CAD build for the part. Positions are in the model's coordinates, mm. Give positions to 0.01 mm unless a question says otherwise; leave off trailing zeros.
```python
from build123d import *

# Parameters (mm, degrees)
BOSS_EXTRUDE1_DEPTH = 749.3
BOSS_EXTRUDE2_DEPTH = 12.7
SKETCH3_W           = 25.4
SKETCH3_H           = 12.7
CUT_EXTRUDE1_DEPTH  = 6.35
SKETCH4_R           = 1.5875
CUT_EXTRUDE2_DEPTH  = 70.358
SKETCH5_R           = 1.5875
CUT_EXTRUDE3_DEPTH  = 70.358


with BuildPart() as part:
    # Sketch1 → Boss-Extrude1 (new body)
    with BuildSketch(Plane.XY):
        Polygon((0, 11.1125), (1.5875, 12.7), (4.7625, 12.7), (6.35, 11.1125), (6.35, 1.5875), (4.7625, 0), (1.5875, 0), (0, 1.5875), align=None)
    extrude(amount=BOSS_EXTRUDE1_DEPTH)

    # Sketch2 → Boss-Extrude2 (add)
    with BuildSketch(Plane.XY.offset(749.3)):
        with BuildLine():
            Line((4.7625, 9.525), (4.7625, 3.175))
            ThreePointArc((4.7625, 3.175), (3.175, 1.5875), (1.5875, 3.175))
            Line((1.5875, 3.175), (1.5875, 9.525))
            ThreePointArc((1.5875, 9.525), (3.175, 11.1125), (4.7625, 9.525))
        make_face()
    extrude(amount=BOSS_EXTRUDE2_DEPTH)

    # Sketch3 → Cut-Extrude1 (cut)
    with BuildSketch(Plane.ZY):
        with Locations((12.7, 6.35)):
            Rectangle(SKETCH3_W, SKETCH3_H)
    extrude(amount=-CUT_EXTRUDE1_DEPTH, mode=Mode.SUBTRACT)

    # Sketch4 → Cut-Extrude2 (cut)
    with BuildSketch(Plane.ZY):
        with BuildLine():
            Line((117.475, 4.7625), (136.525, 4.7625))
            ThreePointArc((136.525, 4.7625), (138.1125, 6.35), (136.525, 7.9375))
            Line((136.525, 7.9375), (117.475, 7.9375))
            ThreePointArc((117.475, 7.9375), (115.8875, 6.35), (117.475, 4.7625))
        make_face()
        with Locations((152.4, 6.35)):
            Circle(SKETCH4_R)
        with BuildLine():
            Line((66.675, 4.7625), (85.725, 4.7625))
            ThreePointArc((85.725, 4.7625), (87.3125, 6.35), (85.725, 7.9375))
            Line((85.725, 7.9375), (66.675, 7.9375))
            ThreePointArc((66.675, 7.9375), (65.0875, 6.35), (66.675, 4.7625))
        make_face()
        with Locations((101.6, 6.35)):
            Circle(SKETCH4_R)
        with BuildLine():
            Line((168.275, 4.7625), (187.325, 4.7625))
            ThreePointArc((187.325, 4.7625), (188.9125, 6.35), (187.325, 7.9375))
            Line((187.325, 7.9375), (168.275, 7.9375))
            ThreePointArc((168.275, 7.9375), (166.6875, 6.35), (168.275, 4.7625))
        make_face()
        with Locations((203.2, 6.35)):
            Circle(SKETCH4_R)
        with BuildLine():
            Line((219.075, 4.7625), (238.125, 4.7625))
            ThreePointArc((238.125, 4.7625), (239.7125, 6.35), (238.125, 7.9375))
            Line((238.125, 7.9375), (219.075, 7.9375))
            ThreePointArc((219.075, 7.9375), (217.4875, 6.35), (219.075, 4.7625))
        make_face()
        with Locations((254, 6.35)):
            Circle(SKETCH4_R)
        with BuildLine():
            Line((269.875, 4.7625), (288.925, 4.7625))
            ThreePointArc((288.925, 4.7625), (290.5125, 6.35), (288.925, 7.9375))
            Line((288.925, 7.9375), (269.875, 7.9375))
            ThreePointArc((269.875, 7.9375), (268.2875, 6.35), (269.875, 4.7625))
        make_face()
        with Locations((304.8, 6.35)):
            Circle(SKETCH4_R)
        with BuildLine():
            Line((320.675, 4.7625), (339.725, 4.7625))
            ThreePointArc((339.725, 4.7625), (341.3125, 6.35), (339.725, 7.9375))
            Line((339.725, 7.9375), (320.675, 7.9375))
            ThreePointArc((320.675, 7.9375), (319.0875, 6.35), (320.675, 4.7625))
        make_face()
        with Locations((355.6, 6.35)):
            Circle(SKETCH4_R)
        with BuildLine():
            Line((371.475, 4.7625), (390.525, 4.7625))
            ThreePointArc((390.525, 4.7625), (392.1125, 6.35), (390.525, 7.9375))
            Line((390.525, 7.9375), (371.475, 7.9375))
            ThreePointArc((371.475, 7.9375), (369.8875, 6.35), (371.475, 4.7625))
        make_face()
        with Locations((406.4, 6.35)):
            Circle(SKETCH4_R)
        with BuildLine():
            Line((422.275, 4.7625), (441.325, 4.7625))
            ThreePointArc((441.325, 4.7625), (442.9125, 6.35), (441.325, 7.9375))
            Line((441.325, 7.9375), (422.275, 7.9375))
            ThreePointArc((422.275, 7.9375), (420.6875, 6.35), (422.275, 4.7625))
        make_face()
        with Locations((457.2, 6.35)):
            Circle(SKETCH4_R)
        with BuildLine():
            Line((473.075, 4.7625), (492.125, 4.7625))
            ThreePointArc((492.125, 4.7625), (493.7125, 6.35), (492.125, 7.9375))
            Line((492.125, 7.9375), (473.075, 7.9375))
            ThreePointArc((473.075, 7.9375), (471.4875, 6.35), (473.075, 4.7625))
        make_face()
        with Locations((508, 6.35)):
            Circle(SKETCH4_R)
        with BuildLine():
            Line((523.875, 4.7625), (542.925, 4.7625))
            ThreePointArc((542.925, 4.7625), (544.5125, 6.35), (542.925, 7.9375))
            Line((542.925, 7.9375), (523.875, 7.9375))
            ThreePointArc((523.875, 7.9375), (522.2875, 6.35), (523.875, 4.7625))
        make_face()
        with Locations((558.8, 6.35)):
            Circle(SKETCH4_R)
        with BuildLine():
            Line((574.675, 4.7625), (593.725, 4.7625))
            ThreePointArc((593.725, 4.7625), (595.3125, 6.35), (593.725, 7.9375))
            Line((593.725, 7.9375), (574.675, 7.9375))
            ThreePointArc((574.675, 7.9375), (573.0875, 6.35), (574.675, 4.7625))
        make_face()
        with Locations((609.6, 6.35)):
            Circle(SKETCH4_R)
        with BuildLine():
            Line((625.475, 4.7625), (644.525, 4.7625))
            ThreePointArc((644.525, 4.7625), (646.1125, 6.35), (644.525, 7.9375))
            Line((644.525, 7.9375), (625.475, 7.9375))
            ThreePointArc((625.475, 7.9375), (623.8875, 6.35), (625.475, 4.7625))
        make_face()
        with Locations((660.4, 6.35)):
            Circle(SKETCH4_R)
        with BuildLine():
            Line((676.275, 4.7625), (695.325, 4.7625))
            ThreePointArc((695.325, 4.7625), (696.9125, 6.35), (695.325, 7.9375))
            Line((695.325, 7.9375), (676.275, 7.9375))
            ThreePointArc((676.275, 7.9375), (674.6875, 6.35), (676.275, 4.7625))
        make_face()
        with Locations((711.2, 6.35)):
            Circle(SKETCH4_R)
        with BuildLine():
            Line((727.075, 4.7625), (746.125, 4.7625))
            ThreePointArc((746.125, 4.7625), (747.7125, 6.35), (746.125, 7.9375))
            Line((746.125, 7.9375), (727.075, 7.9375))
            ThreePointArc((727.075, 7.9375), (725.4875, 6.35), (727.075, 4.7625))
        make_face()
    extrude(amount=-CUT_EXTRUDE2_DEPTH, mode=Mode.SUBTRACT)

    # Sketch5 → Cut-Extrude3 (cut)
    with BuildSketch(Plane.ZY):
        with Locations((50.8, 6.35)):
            Circle(SKETCH5_R)
    extrude(amount=-CUT_EXTRUDE3_DEPTH, mode=Mode.SUBTRACT)


solid = part.part
```
1. Drop flat-ended pins along their axis: pin 1 (7 mm diameter, centred on y = 5.5, z = 753, fed in from -X); pin 2 (1.9 mm diameter, centred on y = 6, z = 758, fed in from +X). Give the stop position or say it passes through.
Responses:
pin 1: stops at x = 1.59
pin 2: stops at x = 4.76
2. Probe line 1 along Y through (x, z) = (4.5, 457); line 2 along Y through (x, z) = (1.5, 326); line 3 along Z through (x, y) = (5.25, 9.25). List the from-to ranges inside material, lowest first.
Responses:
line 1: y = 0 to 4.78, 7.92 to 12.7
line 2: y = 0.09 to 4.76, 7.94 to 12.61
line 3: z = 25.4 to 749.3
3. Saw through at A-A, the plane x = 3.75. Count the separate pieces of the cut face and the enclosed holes in it, and give its area (3 significant figures).
Responses:
separate pieces: 1
enclosed holes: 28
area: 8,240 mm2
